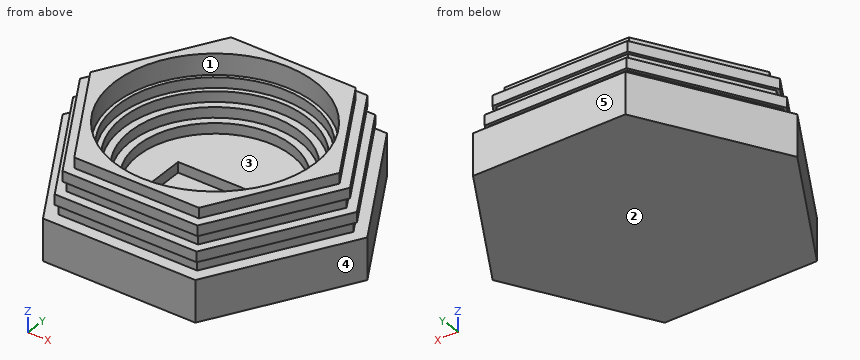
```python
from build123d import *

# Parameters (mm, degrees)
PAD_DEPTH    = 9
SKETCH001_W  = 26.1
SKETCH001_H  = 34.4
POCKET_DEPTH = 3
SKETCH002_R  = 22.22
PAD001_DEPTH = 3
SKETCH003_R  = 24.44
PAD002_DEPTH = 3
SKETCH004_R  = 26.6
PAD003_DEPTH = 3
SKETCH005_R  = 28
PAD004_DEPTH = 3
SKETCH006_R  = 29
PAD005_DEPTH = 3
SKETCH007_R  = 29
PAD006_DEPTH = 3


with BuildPart() as part:
    # Sketch → Pad (new body)
    with BuildSketch(Plane.XY):
        Polygon((44, 0), (22, 38.105118), (-22, 38.105118), (-44, 0), (-22, -38.105118), (22, -38.105118), align=None)
    extrude(amount=PAD_DEPTH)

    # Sketch001 (on Face8 of Pad) → Pocket (cut)
    with BuildSketch(Plane.XY.offset(9)):
        with Locations((0, -13.905118)):
            Rectangle(SKETCH001_W, SKETCH001_H)
    extrude(amount=-POCKET_DEPTH, mode=Mode.SUBTRACT)

    # Sketch002 (on Face5 of Pocket) → Pad001 (join)
    with BuildSketch(Plane.XY.offset(9)):
        Polygon((22, 38.105118), (-22, 38.105118), (-44, 0), (-22, -38.105118), (22, -38.105118), (44, 0), align=None)
        Circle(SKETCH002_R, mode=Mode.SUBTRACT)
    extrude(amount=PAD001_DEPTH)

    # Sketch003 (on Face14 of Pad001) → Pad002 (join)
    with BuildSketch(Plane.XY.offset(12)):
        Polygon((40, 0), (20, 34.641016), (-20, 34.641016), (-40, 0), (-20, -34.641016), (20, -34.641016), align=None)
        Circle(SKETCH003_R, mode=Mode.SUBTRACT)
    extrude(amount=PAD002_DEPTH)

    # Sketch004 (on Face21 of Pad002) → Pad003 (join)
    with BuildSketch(Plane.XY.offset(15)):
        Polygon((41, 0), (20.5, 35.507042), (-20.5, 35.507042), (-41, 0), (-20.5, -35.507042), (20.5, -35.507042), align=None)
        Circle(SKETCH004_R, mode=Mode.SUBTRACT)
    extrude(amount=PAD003_DEPTH)

    # Sketch005 (on Face28 of Pad003) → Pad004 (join)
    with BuildSketch(Plane.XY.offset(18)):
        Polygon((19, 32.908965), (-19, 32.908965), (-38, 0), (-19, -32.908965), (19, -32.908965), (38, 0), align=None)
        Circle(SKETCH005_R, mode=Mode.SUBTRACT)
    extrude(amount=PAD004_DEPTH)

    # Sketch006 (on Face35 of Pad004) → Pad005 (join)
    with BuildSketch(Plane.XY.offset(21)):
        Polygon((39, 0), (19.5, 33.774991), (-19.5, 33.774991), (-39, 0), (-19.5, -33.774991), (19.5, -33.774991), align=None)
        Circle(SKETCH006_R, mode=Mode.SUBTRACT)
    extrude(amount=PAD005_DEPTH)

    # Sketch007 (on Face42 of Pad005) → Pad006 (join)
    with BuildSketch(Plane.XY.offset(24)):
        Polygon((36, 0), (18, 31.176915), (-18, 31.176915), (-36, 0), (-18, -31.176915), (18, -31.176915), align=None)
        Circle(SKETCH007_R, mode=Mode.SUBTRACT)
    extrude(amount=PAD006_DEPTH)


solid = part.part
```
Geometry check sheet. Reference: the model listing, model coordinates, mm. Face numbers are marked on the shaded views. A direction names the side the tool comes from. Give positions to 0.01 mm unless a question says otherwise; leave off trailing zeros. Order: outer loops, then holes, each group sorted by start corner. A loop starts at its lowest first (then second) coordinate and runs counter-clockwise, first axis right, second up. Notation, with made-up numbers: (23.5, -31) - (43.5, -31) arc R12 ccw to (43.5, -27) - close; hole circle Ø6 at (-40, -29.5). An arc over 180 degrees is marked (long way). Answer in a Markdown table with one row per item. Add a question column.
Q1. Gauge pin test, flat ends, axial feed: pin 1 (1 mm diameter, centred on x = 12.5, z = 23.5, fed in from +Y) (3 decimals); pin 2 (6 mm diameter, centred on x = 34, y = -18, fed in from +Z); pin 3 (1.5 mm diameter, centred on x = -1, z = 19.5, fed in from +Y). Record the tip position at first contact, or that the pin passes through.
Q2. Material ranges on probe 1 along Y at (x, z) = (0, 12.9); probe 2 along Z at (x, y) = (-22, -32.5); probe 3 along Y at (x, z) = (0, 19), recorded low to high. Write a range as from..to.
Q3. Tool access check on the marked faces 1 and 2. Record the directions out of +Z, -Z, +X, -X, +Y, -Y that give a thin tool (end or side, any length) a straight path to the whole face; none if there is none.
Q4. Cross-section at B-B, the plane z = 2.25. Enter the section's corners in (x, y), then the cut area to 3 significant figures.
Q5. Cross-section at A-A, the plane z = 19. Enter the section's corners in (x, y), then the cut area to 3 significant figures.
Q6. Mould release check, pull along X, two halves, no side actions. Record for the marked faces 3, 4 and 5: pulls with the +X half, pulls with the -X half, needs draft (parallel to the pull), parting line crosses it, or undercut.
Check values:
| question | item | result |
|---|---|---|
| 1 | pin 1 | stops at y = 33.775 |
| 1 | pin 2 | stops at z = 18 |
| 1 | pin 3 | stops at y = 32.91 |
| 2 | probe 1 | y = -34.64..-24.44, 24.44..34.64 |
| 2 | probe 2 | z = 0..12, 15..18 |
| 2 | probe 3 | y = -32.91..-28, 28..32.91 |
| 3 | face 1 | +Z |
| 3 | face 2 | -Z, +X, -X, +Y, -Y |
| 4 | outline | (-44, 0) - (-22, -38.11) - (22, -38.11) - (44, 0) - (22, 38.11) - (-22, 38.11) - close |
| 4 | area | 5,030 mm^2 |
| 5 | outline | (-38, 0) - (-19, -32.91) - (19, -32.91) - (38, 0) - (19, 32.91) - (-19, 32.91) - close; hole circle Ø56 at (0, 0) |
| 5 | area | 1,290 mm^2 |
| 6 | face 3 | undercut |
| 6 | face 4 | pulls with the +X half |
| 6 | face 5 | needs draft |
